Geometry: final body of the model. Coordinates: model frame, mm. Face numbers are marked on the shaded views. A direction names the side the tool comes from. Round coordinates to 2 decimals unless told otherwise and drop trailing zeros. Order: outer loops, then holes, each group sorted by start corner. A loop starts at its lowest first (then second) coordinate and runs counter-clockwise, first axis right, second up. Notation, with made-up numbers: M -4.5,8.25 L 19.5,8.25 A19 cw 19.5,19.25 Z; hole C 15.25,83 d7. An arc over 180 degrees is marked long. Return JSON: item names as keys, results as strings. Group by question number.
Q1. Ray query, probe 1 along Z at (x, y) = (5, 2.7); probe 2 along Z at (x, y) = (12, 2.95); probe 3 along X at (y, z) = (2.6, -8). Return the intervals inside material, ascending.
Q2. Cut plane A-A on x = 70. Output: boundary loops of the cut face in (y, z).
Q3. Cut plane B-B on x = 46.5. Output: boundary loops of the cut face in (y, z).
Q4. Access query for the marked faces 1 and 2. Directions: +Z, -Z, +X, -X, +Y, -Y. A direction counts if a zero-diameter tool reaches every point of the face in a straight line with its end or side. Return the directions, or none.
Q5. Contact query for flat-ended pins moving along their axis: pin 1 (3 mm diameter, centred on x = 4.5, z = -10, fed in from +Y); pin 2 (0.6 mm diameter, centred on y = 2.5, z = -4, fed in from +X); pin 3 (0.8 mm diameter, centred on x = 5.5, z = -2, fed in from +Y); pin 4 (10 mm diameter, centred on x = 43.5, z = -21.5, fed in from -Y). Output: stop coordinate, or through.
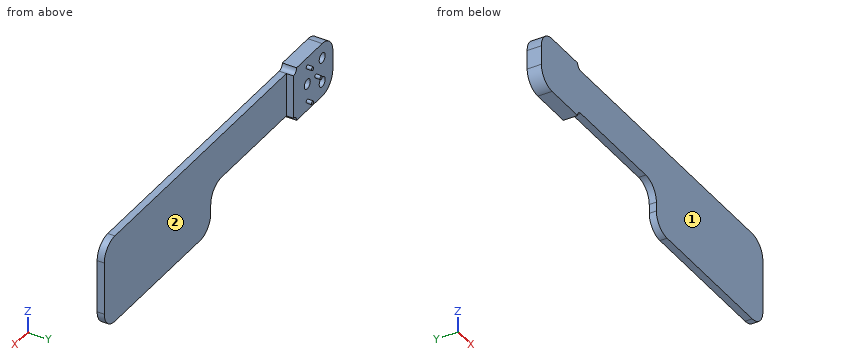
```python
from build123d import *

# Parameters (mm, degrees)
SKETCH_1_W          = 17
SKETCH_1_H          = 12.4
EXTRUDE_1_DEPTH     = 4
SKETCH_2_R          = 1.4
CUT_EXTRUDE_1_DEPTH = 3
SKETCH_3_W          = 12.4
SKETCH_3_H          = 2
EXTRUDE_2_DEPTH     = 37
SKETCH_4_W          = 17
SKETCH_4_H          = 1.5
EXTRUDE_3_DEPTH     = 4
FILLET_1_R          = 5
SKETCH_5_R          = 0.5
EXTRUDE_4_DEPTH     = 1.5
EXTRUDE_5_DEPTH     = 2
SKETCH_7_W          = 50
SKETCH_7_H          = 25
EXTRUDE_6_DEPTH     = 2
FILLET_2_R          = 5
FILLET_3_R          = 5
EXTRUDE_7_DEPTH     = 2


with BuildPart() as part:
    # 草图1 → 凸台-拉伸1 (new body)
    with BuildSketch(Plane(origin=(0, 0, 0), x_dir=(1, 0, 0), z_dir=(0, 1, 0))):
        with Locations((8.5, 6.2)):
            Rectangle(SKETCH_1_W, SKETCH_1_H)
    extrude(amount=EXTRUDE_1_DEPTH)

    # 草图2 → 切除-拉伸1 (cut)
    with BuildSketch(Plane(origin=(0, 4, 0), x_dir=(1, 0, 0), z_dir=(0, 1, 0))):
        with Locations((12, 6.2)):
            Circle(SKETCH_2_R)
        with Locations((5, 9.7)):
            Circle(SKETCH_2_R)
        with Locations((5, 2.7)):
            Circle(SKETCH_2_R)
    extrude(amount=-CUT_EXTRUDE_1_DEPTH, mode=Mode.SUBTRACT)

    # 草图3 → 凸台-拉伸2 (add)
    with BuildSketch(Plane(origin=(17, 0, 0), x_dir=(0, 0, -1), z_dir=(1, 0, 0))):
        with Locations((6.2, 1)):
            Rectangle(SKETCH_3_W, SKETCH_3_H)
    extrude(amount=EXTRUDE_2_DEPTH)

    # 草图4 → 凸台-拉伸3 (add)
    with BuildSketch(Plane(origin=(0, 4, 0), x_dir=(1, 0, 0), z_dir=(0, 1, 0))):
        with Locations((8.5, 13.15)):
            Rectangle(SKETCH_4_W, SKETCH_4_H)
        with Locations((8.5, -0.75)):
            Rectangle(SKETCH_4_W, SKETCH_4_H)
    extrude(amount=-EXTRUDE_3_DEPTH)

    # 圆角1
    fillet_1_edges = [part.edges().sort_by_distance(p)[0] for p in [
        (0, 2, -13.9),
        (0, 2, 1.5),
    ]]
    fillet(fillet_1_edges, radius=FILLET_1_R)

    # 草图5 → 凸台-拉伸4 (add)
    with BuildSketch(Plane(origin=(0, 4, 0), x_dir=(1, 0, 0), z_dir=(0, 1, 0))):
        with Locations((8, 6.2)):
            Circle(SKETCH_5_R)
        with Locations((12, 11.2)):
            Circle(SKETCH_5_R)
        with Locations((12, 1.2)):
            Circle(SKETCH_5_R)
    extrude(amount=EXTRUDE_4_DEPTH)

    # 草图6 → 凸台-拉伸5 (add)
    with BuildSketch(Plane(origin=(0, 2, 0), x_dir=(1, 0, 0), z_dir=(0, 1, 0))):
        with BuildLine():
            Line((17, 13.9), (17, 12.4))
            Line((17, 12.4), (18.5, 12.4))
            ThreePointArc((18.5, 12.4), (17.439339828, 12.839339828), (17, 13.9))
        make_face()
        with BuildLine():
            Line((17, -1.5), (17, 0))
            Line((17, 0), (18.5, 0))
            ThreePointArc((18.5, 0), (17.439339828, -0.439339828), (17, -1.5))
        make_face()
    extrude(amount=-EXTRUDE_5_DEPTH)

    # 草图7 → 凸台-拉伸6 (add)
    with BuildSketch(Plane.XZ):
        with Locations((79, -12.5)):
            Rectangle(SKETCH_7_W, SKETCH_7_H)
    extrude(amount=-EXTRUDE_6_DEPTH)

    # 圆角2
    fillet_2_edges = [part.edges().sort_by_distance(p)[0] for p in [
        (54, 1, -25),
        (54, 1, -12.4),
    ]]
    fillet(fillet_2_edges, radius=FILLET_2_R)

    # 圆角3
    fillet_3_edges = [part.edges().sort_by_distance(p)[0] for p in [
        (104, 1, 0),
        (104, 1, -25),
    ]]
    fillet(fillet_3_edges, radius=FILLET_3_R)

    # 草图8 → 凸台-拉伸7 (add)
    with BuildSketch(Plane(origin=(0, 2, 0), x_dir=(1, 0, 0), z_dir=(0, 1, 0))):
        with BuildLine():
            Line((18.5, 0), (18.5, 12.4))
            ThreePointArc((18.5, 12.4), (17.439339828, 12.839339828), (17, 13.9))
            Line((17, 13.9), (17, -1.5))
            ThreePointArc((17, -1.5), (17.439339828, -0.439339828), (18.5, 0))
        make_face()
    extrude(amount=EXTRUDE_7_DEPTH)


solid = part.part
```
Result sheet:
{
 "1": {"probe 1": "z = -13.9 to -11.1, -8.3 to -4.1, -1.3 to 1.5", "probe 2": "z = -13.9 to -7.6, -4.8 to 1.5", "probe 3": "x = 0 to 18.5"},
 "2": {"outline": "M 0,-25 L 2,-25 L 2,0 L 0,0 Z"},
 "3": {"outline": "M 0,-12.4 L 2,-12.4 L 2,0 L 0,0 Z"},
 "4": {"face 1": "+Z, -Z, +X, -X, -Y", "face 2": "+Z, -Z, +X, +Y"},
 "5": {"pin 1": "stops at y = 4", "pin 2": "stops at x = 18.5", "pin 3": "stops at y = 1", "pin 4": "passes through"}
}
